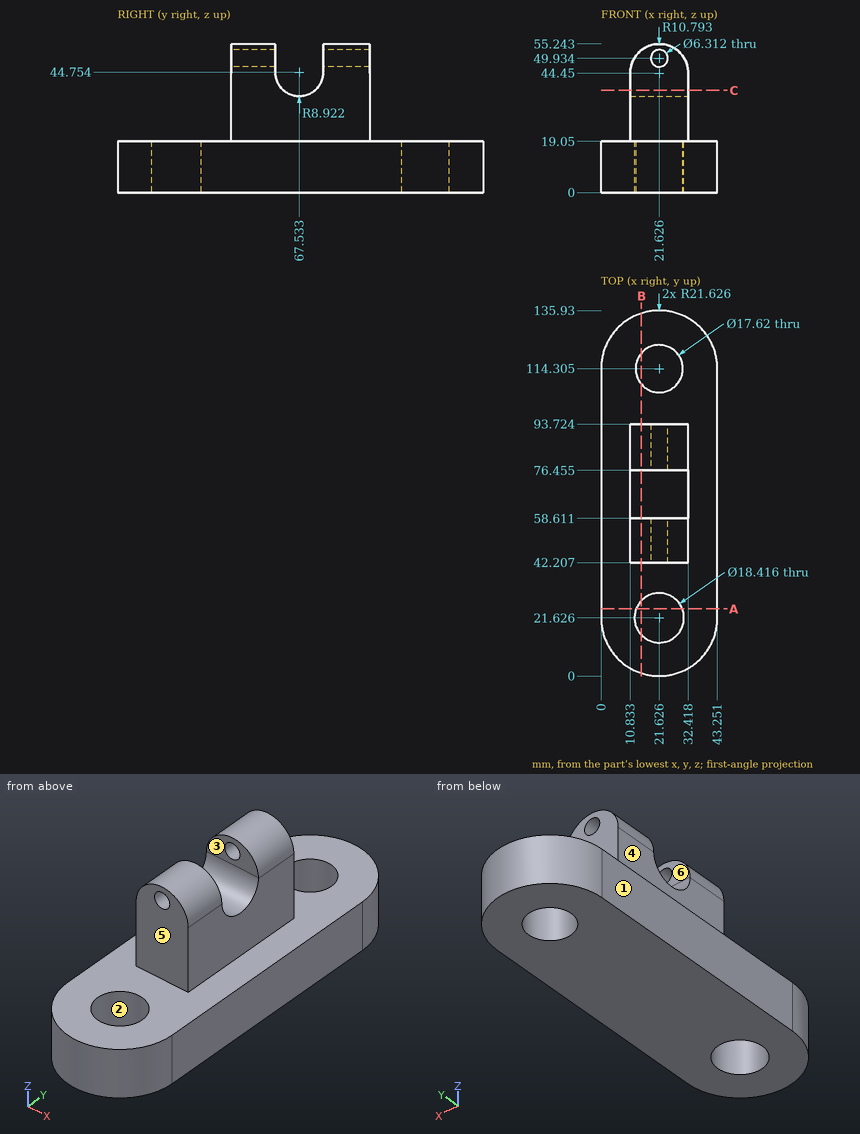
Can you work these out from the drawing? Everything is in mm from the part's minimum corner. A direction names the side the tool comes from. Round coordinates to 2 decimals unless told otherwise and drop trailing zeros. Order: outer loops, then holes, each group sorted by start corner. A loop starts at its lowest first (then second) coordinate and runs counter-clockwise, first axis right, second up. Notation, with made-up numbers: M 29,25 L 73,25 A32 ccw 73,62 Z; hole C 63,9.5 d4. An arc over 180 degrees is marked long. One line per question, with ' | ' between items.
1) If we mould it in two halves opening along X, with no side actions, what happens to the marked faces 1, 2 and 3? For each: +X half, -X half, draft (parallel to the pull), parting line (faces both ways), or undercut.
Working result:
face 1: -X half | face 2: undercut | face 3: draft
2) I want a section at A-A, the plane y = 25. Write out the boundary of the cut face in (x, z).
Working result:
outline: M 0,0 L 13.06,0 L 13.06,19.05 L 0,19.05 Z; M 30.19,0 L 43.25,0 L 43.25,19.05 L 30.19,19.05 Z
3) For pin 1 Ø5 at (y, z) = (16.5, 10) entering from -X; pin 2 Ø3 at (y, z) = (81.5, 26.5) entering from -X; pin 3 Ø10 at (x, z) = (28, 38.5) entering from -Y; pin 4 Ø4 at (x, z) = (21.63, 49.93) entering from +Y, each with a flat end and sliding along its axis, tell me the tip position at first contact or that it passes through.
Working result:
pin 1: x = 0.16 | pin 2: x = 10.83 | pin 3: y = 42.21 | pin 4: through
4) I need wall thicknesses on line 1 along Z through (x, y) = (40, 34); line 2 along X through (y, z) = (93, 24.5); line 3 along Z through (x, y) = (31, 74) (1 decimal). Which ranges of each line are inside material? Lowest first, please.
Working result:
line 1: 0 to 19.05 | line 2: 10.83 to 32.42 | line 3: 0 to 38.6
5) I want a section at B-B, the plane x = 15. State how many separate pieces and enclosed holes the cut face has, then the cut area to 3 significant figures.
Working result:
separate pieces: 3 | enclosed holes: 0 | area: 3,560 mm²
6) I want a section at C-C, the plane z = 38. Write out the boundary of the cut face in (x, y).
Working result:
outline: M 10.83,42.21 L 32.42,42.21 L 32.42,61.7 L 10.83,61.7 Z; M 10.83,73.36 L 32.42,73.36 L 32.42,93.72 L 10.83,93.72 Z
7) For the marked faces 4, 5 and 6, which set-ups out of +Z, -Z, +X, -X, +Y, -Y let a thin tool reach every point of the face, with its end or its side?
Working result:
face 4: +Z, -X, +Y, -Y | face 5: +Z, +X, -X, -Y | face 6: +Z, +X, -X
